Input: part model. Units: mm. Frame: model coordinates. A direction names the side the tool comes from. Coordinates: 2 decimals unless noted, no trailing zeros. Loops run counter-clockwise (first coordinate to the right, second up) from the corner with the lowest first, then second, coordinate; pieces in that order, holes last. Notation, with made-up numbers: (70.25, -26) - (78.25, -26) arc R15 cw to (78.25, -14) - close; hole circle Ø2 at (45.25, 68.5). An arc over 180 degrees is marked (long way). Answer as CSV lines item,"result". Start each with the question number.
```python
from build123d import *

# Parameters (mm, degrees)
F0_R     = 9.46522
F3_DEPTH = 1
F1_R     = 3.950475
F4_DEPTH = 9
F2_R     = 2.248498
F6_DEPTH = 9
F5_R     = 2.248498
F7_DEPTH = 1


with BuildPart() as f3:
    # F0 (on Top) → F3 (new body)
    with BuildSketch(Plane.XY):
        Circle(F0_R)
    extrude(amount=F3_DEPTH)

    # F1 (on Top) → F4 (join)
    with BuildSketch(Plane.XY):
        Circle(F1_R)
    extrude(amount=F4_DEPTH)

    # F2 (on Top) → F6 (cut)
    with BuildSketch(Plane.XY):
        Circle(F2_R)
    extrude(amount=F6_DEPTH, mode=Mode.SUBTRACT)

    # F5 (on Top) → F7 (join)
    with BuildSketch(Plane.XY):
        Circle(F5_R)
    extrude(amount=F7_DEPTH)


solid = f3.part
```
Item 1: Material intervals for probe 1 along Y at (x, z) = (0, 7); probe 2 along Z at (x, y) = (-5.5, 3.25); probe 3 along Y at (x, z) = (1, 5), sorted ascending.
Item 2: Section query C-C, the plane z = 8. Output: boundary loops of the cut face in (x, y).
Item 3: Draft query along X for faces 3 (the cylindrical face through (3.768, 1.187, 4.944)), 4 (the flat face through (2, -2, 9)), 5 (the flat face through (0, 0, 1)). Return one class per face: pulls with the +X half, pulls with the -X half, needs draft (parallel to the pull), parting line crosses it, or undercut.
Item 4: Section query D-D, the plane x = -2.5. Output: boundary loops of the cut face in (y, z).
Item 5: Section query A-A, the plane y = 0. Output: boundary loops of the cut face in (x, z).
Item 6: Set-up query: faces 1 (the cylindrical face through (-9.456, 0.416, 0.493)), 2 (the flat face through (4.1, 0.1, 1)). Return all of +Z, -Z, +X, -X, +Y, -Y with unobstructed straight access to the full face (end or side cutting, diameter ignored); none if empty.
Item 7: Contact query for flat-ended pins moving along their axis: P1, Ø8, axis at x = -7.5, y = -2, coming from the -Z side; P2, Ø5, axis at x = 4, z = 4.5, coming from the +Y side; P3, Ø2, axis at y = 4.5, z = 6, coming from the -X side; P4, Ø3.5, axis at x = 0, y = 0, coming from the +Z side. Output: stop coordinate, or through.
Response values:
1,probe 1,"y = -3.95 to -2.25, 2.25 to 3.95"
1,probe 2,"z = 0 to 1"
1,probe 3,"y = -3.82 to -2.01, 2.01 to 3.82"
2,outline,"circle Ø7.9 at (0, 0); hole circle Ø4.5 at (0, 0)"
3,face 3,"parting line crosses it"
3,face 4,"needs draft"
3,face 5,"undercut"
4,outline,"(-9.13, 0) - (9.13, 0) - (9.13, 1) - (3.06, 1) - (3.06, 9) - (-3.06, 9) - (-3.06, 1) - (-9.13, 1) - close"
5,outline,"(-9.47, 0) - (9.47, 0) - (9.47, 1) - (3.95, 1) - (3.95, 9) - (2.25, 9) - (2.25, 1) - (-2.25, 1) - (-2.25, 9) - (-3.95, 9) - (-3.95, 1) - (-9.47, 1) - close"
6,face 1,"+Z, -Z"
6,face 2,"+Z"
7,P1,"stops at z = 0"
7,P2,"stops at y = 3.65"
7,P3,"stops at x = -1.83"
7,P4,"stops at z = 1"
